Design review of the part built by this model. Coordinates are the model's own, in mm. Face numbers are marked on the shaded views. A direction names the side the tool comes from. Coordinates: 2 decimals unless noted, no trailing zeros. Write each loop counter-clockwise with the first axis right and the second up, starting at its lowest first coordinate (ties: lowest second). Pieces come first, ordered by that corner, then holes.
Q1. For L1, parallel to Y at x = 16.75, z = -1.5; L2, parallel to X at y = 14.25, z = -7.5; L3, parallel to Z at x = 1.25, y = 17.5, list the stretches that pass through material, from the lowest coordinate up.
Q2. Take a section at C-C, the plane y = 10. Write out the cut boundary in (x, z).
Q3. Take a section at D-D, the plane x = 17.25. Write out the cut boundary in (y, z), plus the area to 3 significant figures.
Q4. For the marked faces 1, 2, 3 and 4, list the 3-axis set-ups (+Z, -Z, +X, -X, +Y, -Y) from which the entire face can be reached by the end or side of a thin tool; tool diameter is ignored.
Q5. For pin 1 Ø6 at (x, y) = (6, 11.5) entering from -Z; pin 2 Ø6 at (x, y) = (12, 4) entering from +Z; pin 3 Ø5 at (x, y) = (16.5, 8) entering from +Z, all flat-tipped, find the tip position at first contact; note any pin that passes through.
Q6. Take a section at A-A, the plane z = -7.5. Write out the cut boundary in (x, y), plus the area to 3 significant figures.
Q7. Take a section at B-B, the plane x = 11.5. Write out the cut boundary in (y, z).
Q8. The part is to be moulded in two halves that separate along Y. For the marked faces 5, 6, 7 and 8, say which applies: released by +Y, released by -Y, zero draft, split by the parting line, or undercut.
Autodesk Fusion 360 part; units mm, degrees
sketch "Sketch1" plane through (0, 0, 0) normal (0, 1, 0) x (1, 0, 0)
  line L0 (0, 0) -> (23, 0)
  line L1 (23, 0) -> (23, 27)
  line L2 (23, 27) -> (0, 27)
  line L3 (0, 27) -> (0, 0)
  line L4 (11.5, 0) -> (11.5, 27)
  line L5 (11.5, 0) -> (11.5, 6)
  line L6 (23, 6) -> (0, 6)
  line L7 (11.5, 6) -> (11.5, 10)
  line L8 (0, 6) -> (23, 6)
  line L9 (23, 6) -> (23, 10)
  line L10 (23, 10) -> (0, 10)
  line L11 (0, 10) -> (0, 6)
  dimension "d1" = 23
  dimension "d2" = 27
  dimension "d3" = 6
  dimension "d4" = 4
extrude "Extrude1" add sketch "Sketch1" along normal blind 4
sketch "Sketch2" plane through (0, 4, 0) normal (0, 1, 0) x (-1, 0, 0)
  line L0 (0, -27) -> (0, 0)
  line L1 (0, 0) -> (-23, 0)
  line L2 (-23, 0) -> (-23, -27)
  line L3 (-23, -27) -> (0, -27)
  line L4 (-11.5, 0) -> (-11.5, -6)
  line L5 (-23, -6) -> (0, -6)
  line L6 (0, -6) -> (0, -10)
  line L7 (0, -6) -> (-23, -6)
  line L8 (-23, -10) -> (-23, -6)
  line L9 (-23, -10) -> (0, -10)
  dimension "d7" = 6
  dimension "d8" = 4
extrude "Extrude2" add sketch "Sketch2" along normal blind 23 contours L0 L2 L5 L6 L7 L8 L9
sketch "Sketch3" plane through (0, 0, -6) normal (0, 0, 1) x (1, 0, 0)
  line L0 (0, 4) -> (23, 4)
  line L1 (23, 4) -> (23, 27)
  line L2 (23, 27) -> (0, 27)
  line L3 (0, 27) -> (0, 4)
  line L4 (11.5, 0) -> (11.5, 19)
  circle A0 centre (11.5003, 15.35) radius 3.65
  line L5 (15.1503, 15.35) -> (15.1503, 4)
  line L6 (7.8503, 4) -> (7.8503, 15.35)
  dimension "d11" = 19
  dimension "d12" = 7.3
extrude "Extrude5" cut sketch "Sketch3" against normal blind 4 contours L0 L4 A0 L6 | L0 L4 A0 L5 | L4 A0 | L4 A0
sketch "Sketch4" plane through (0, 27, 0) normal (0, 1, 0) x (-1, 0, 0)
  line L0 (0, -6) -> (-23, -6)
  line L1 (-23, -6) -> (-23, -10)
  line L2 (-23, -10) -> (0, -10)
  line L3 (0, -10) -> (0, -6)
  circle A0 centre (-11.5, -10) radius 1.6
  dimension "d15" = 3.2
extrude "Extrude4" cut sketch "Sketch4" against normal blind 9 contours L2 A0 picked at (-11.109, -9.6372)
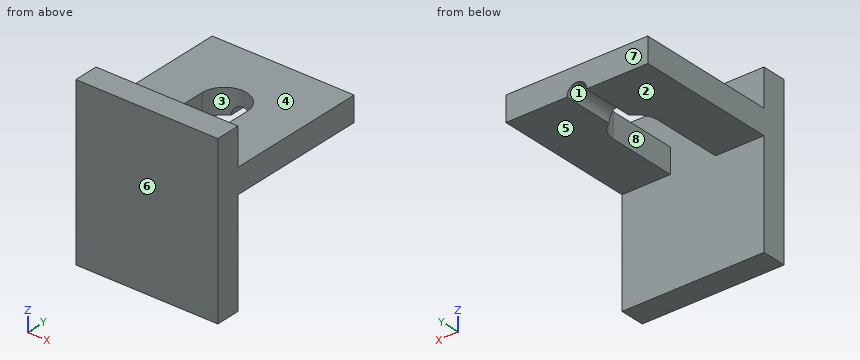
Responses:
1. L1: y = 0 to 4
1. L2: x = 0 to 7.85, 15.15 to 23
1. L3: z = -10 to -6
2. outline: (0, -10) - (7.85, -10) - (7.85, -6) - (0, -6) - close; (15.15, -10) - (23, -10) - (23, -6) - (15.15, -6) - close
3. outline: (0, -27) - (4, -27) - (4, -10) - (27, -10) - (27, -6) - (4, -6) - (4, 0) - (0, 0) - close
3. area: 200 mm2
4. face 1: -Z, +Y
4. face 2: -Z, +X, -X, +Y
4. face 3: +Z, -Z
4. face 4: +Z, +X, -X, +Y
5. pin 1: stops at z = -10
5. pin 2: stops at z = 0
5. pin 3: stops at z = -6
6. outline: (0, 0) - (23, 0) - (23, 27) - (0, 27) - close; hole (7.85, 4) - (15.15, 4) - (15.15, 15.35) arc R3.65 ccw to (7.85, 15.35) - close
6. area: 517 mm2
7. outline: (0, -27) - (4, -27) - (4, 0) - (0, 0) - close; (19, -8.4) - (27, -8.4) - (27, -6) - (19, -6) - close
8. face 5: zero draft
8. face 6: released by -Y
8. face 7: released by +Y
8. face 8: undercut
